Geometry check sheet. Reference: the model listing, model coordinates, mm. A direction names the side the tool comes from. Round coordinates to 2 decimals unless told otherwise and drop trailing zeros. Loops run counter-clockwise (first coordinate to the right, second up) from the corner with the lowest first, then second, coordinate; pieces in that order, holes last.
```python
from build123d import *

# Parameters (mm, degrees)
F0_W     = 60.1664371789
F0_H     = 61.1762590706
F1_DEPTH = 63.5
F2_T     = -5.08
F3_R     = 19.05
F4_DEPTH = 61.1762590706
F5_R     = 38.1
F7_R     = 25.4


# Not quite as in the source:
# - a feature of the source that left no trace in its solid (it failed there, or was rolled back) is left out


with BuildPart() as f1:
    # F0 (on Top) → F1 (new body)
    with BuildSketch(Plane.XY):
        Rectangle(F0_W, F0_H)
    extrude(amount=F1_DEPTH)

    # F2
    f2_openings = [f1.faces().sort_by_distance(p)[0] for p in [
        (30.083219, 0, 31.75),
        (0, 0, 63.5),
    ]]
    offset(amount=F2_T, openings=f2_openings)

    # F3 (on face) → F4 (cut, through all)
    with BuildSketch(Plane(origin=(0, 30.5881295353, 0), x_dir=(-1, 0, 0), z_dir=(0, 1, 0))):
        with Locations((0, 31.75)):
            Circle(F3_R)
    extrude(amount=-F4_DEPTH, mode=Mode.SUBTRACT)

    # F5
    f5_edges = [f1.edges().sort_by_distance(p)[0] for p in [
        (30.083219, -28.04813, 63.5),
        (30.083219, 28.04813, 63.5),
    ]]
    fillet(f5_edges, radius=F5_R)

    # F7
    f7_edges = [f1.edges().sort_by_distance(p)[0] for p in [
        (-30.083219, 0, 0),
        (-25.003219, 0, 5.08),
    ]]
    fillet(f7_edges, radius=F7_R)


solid = f1.part
```
1) Sectioned sample at B-B, the plane z = 27. Record the cut outline in (x, y).
Report:
outline: (-30.08, -30.59) - (-18.45, -30.59) - (-18.45, -25.51) - (-24.76, -25.51) - (-24.76, 25.51) - (-18.45, 25.51) - (-18.45, 30.59) - (-30.08, 30.59) - close; (18.45, -30.59) - (30.05, -30.59) - (30.05, -25.51) - (18.45, -25.51) - close; (18.45, 25.51) - (30.05, 25.51) - (30.05, 30.59) - (18.45, 30.59) - close
2) Gauge pin test, flat ends, axial feed: pin 1 (8 mm diameter, centred on y = 3.5, z = 49.5, fed in from +X); pin 2 (5 mm diameter, centred on x = -10.5, y = -8, fed in from +Z); pin 3 (10 mm diameter, centred on x = -8.5, y = 12, fed in from +Z). Record the tip position at first contact, or that the pin passes through.
Report:
pin 1: stops at x = -25
pin 2: stops at z = 8.9
pin 3: stops at z = 9.22
3) Sectioned sample at C-C, the plane x = 10. Record the cut outline in (y, z).
Report:
outline: (-30.59, 0) - (30.59, 0) - (30.59, 15.54) - (25.51, 15.54) - (25.51, 5.08) - (-25.51, 5.08) - (-25.51, 15.54) - (-30.59, 15.54) - close; (-30.59, 47.96) - (-25.51, 47.96) - (-25.51, 58.97) - (-30.59, 58.97) - close; (25.51, 47.96) - (30.59, 47.96) - (30.59, 58.97) - (25.51, 58.97) - close
4) Sectioned sample at D-D, the plane y = -17. Record the cut outline in (x, z).
Report:
outline: (-30.08, 25.4) arc R25.4 ccw to (-4.68, 0) - (30.08, 0) - (30.08, 5.08) - (0.4, 5.08) arc R25.4 cw to (-25, 30.48) - (-25, 63.5) - (-30.08, 63.5) - close
5) Access from +Z, -Z, +X, -X, +Y, -Y to the whole of each face (thin tool, end or side, straight path). Record for faces 1 (the face through (21, 25.508, 34)), 2 (the face through (12, 0, 0)).
Report:
face 1: +Z, +X
face 2: -Z, +X, -X, +Y, -Y
6) Mould release check, pull along X, two halves, no side actions. Record for faces 3 (the face through (-14, -30.588, 17)), 4 (the face through (2.48, -28.013, 50.638)), 5 (the face through (-30.083, 0, 44)): +X half, -X half, draft (parallel to the pull), parting line (faces both ways), or undercut.
Report:
face 3: draft
face 4: undercut
face 5: -X half
7) Sectioned sample at A-A, the plane y = 26.5. Record the cut outline in (x, z), then the cut area to 3 significant figures.
Report:
outline: (-30.08, 25.4) arc R25.4 ccw to (-4.68, 0) - (30.08, 0) - (30.08, 25.4) arc R38.1 ccw to (-8.02, 63.5) - (-30.08, 63.5) - close; hole circle Ø38.1 at (0, 31.75)
area: 2,230 mm2
8) Scan lines: line 1 along Y through (x, z) = (22.5, 21.5); line 2 along Z through (x, y) = (0, 26.9); line 3 along X through (y, z) = (-29, 31). Record each from-to range of solid material in increasing order.
Report:
line 1: y = -30.59 to -25.51, 25.51 to 30.59
line 2: z = 0 to 12.7, 50.8 to 62.65
line 3: x = -30.08 to -19.04, 19.04 to 29.67
